Input: part model. Units: mm. Frame: model coordinates. A direction names the side the tool comes from. Round coordinates to 2 decimals unless told otherwise and drop trailing zeros. Write each loop counter-clockwise with the first axis right and the second up, starting at its lowest first coordinate (ties: lowest second). Pieces come first, ordered by that corner, then holes. Notation, with made-up numbers: (27, -12) - (43, -12) arc R27 ccw to (43, 8) - close; hole circle Ø9 at (43, -10). An arc over 180 degrees is marked (long way). Use one line per item in the form item = value.
```python
from build123d import *

# Parameters (mm, degrees)
BOSS_EXTRUDE1_DEPTH     = 60
SKETCH2_W               = 95.474406292
SKETCH2_H               = 38.1
SKETCH2_R               = 1.55
BOSS_EXTRUDE2_DEPTH     = 5.08
SKETCH4_R               = 1.8
CUT_EXTRUDE1_DEPTH      = 96.52
CUT_EXTRUDE1_DEPTH_BACK = 107.696


with BuildPart() as part:
    # Sketch1 → Boss-Extrude1 (new body)
    with BuildSketch(Plane(origin=(0, 0, 0), x_dir=(1, 0, 0), z_dir=(0, 1, 0))):
        with BuildLine():
            Line((-25.4, -19.05), (25.4, -19.05))
            ThreePointArc((25.4, -19.05), (44.45, 0), (25.4, 19.05))
            Line((25.4, 19.05), (-25.4, 19.05))
            ThreePointArc((-25.4, 19.05), (-44.45, 0), (-25.4, -19.05))
        make_face()
        with BuildLine():
            Line((-25.4, -13.97), (25.4, -13.97))
            ThreePointArc((25.4, -13.97), (39.37, 0), (25.4, 13.97))
            Line((25.4, 13.97), (-25.4, 13.97))
            ThreePointArc((-25.4, 13.97), (-39.37, 0), (-25.4, -13.97))
        make_face(mode=Mode.SUBTRACT)
    extrude(amount=BOSS_EXTRUDE1_DEPTH)

    # Sketch2 → Boss-Extrude2 (add)
    with BuildSketch(Plane(origin=(0, 60, 0), x_dir=(1, 0, 0), z_dir=(0, 1, 0))):
        Rectangle(SKETCH2_W, SKETCH2_H)
        with Locations((43.019742204, 15.162081353)):
            Circle(SKETCH2_R, mode=Mode.SUBTRACT)
        with Locations((43.019742204, -15.162081353)):
            Circle(SKETCH2_R, mode=Mode.SUBTRACT)
        with Locations((-43.019742204, -15.162081353)):
            Circle(SKETCH2_R, mode=Mode.SUBTRACT)
        with Locations((-43.019742204, 15.162081353)):
            Circle(SKETCH2_R, mode=Mode.SUBTRACT)
    extrude(amount=-BOSS_EXTRUDE2_DEPTH)

    # Sketch4 → Cut-Extrude1 (cut, two sides)
    with BuildSketch(Plane(origin=(0, 0, 0), x_dir=(0, 0, -1), z_dir=(1, 0, 0))) as cut_extrude1_sk:
        with Locations((0, 5.08)):
            Circle(SKETCH4_R)
    extrude(amount=CUT_EXTRUDE1_DEPTH, mode=Mode.SUBTRACT)
    extrude(cut_extrude1_sk.sketch, amount=-CUT_EXTRUDE1_DEPTH_BACK, mode=Mode.SUBTRACT)


solid = part.part
```
(1) Draft query along Y for faces 1 (the face through (-1, 60, 0)), 2 (the face through (41.815, 3.323, 0.39)), 3 (the face through (-41.815, 3.323, 0.39)), 4 (the face through (44.5, 57.5, 14.7)). Return one class per face: released by +Y, released by -Y, zero draft, split by the parting line, or undercut.
Derived:
face_1 = released by +Y
face_2 = undercut
face_3 = undercut
face_4 = zero draft
(2) Material intervals for L1, parallel to Z at x = -21, y = 43; L2, parallel to X at y = 42, z = 0.5; L3, parallel to Y at x = 16.5, z = 8.5, sorted ascending.
Derived:
L1 = -19.05 to -13.97, 13.97 to 19.05
L2 = -44.44 to -39.36, 39.36 to 44.44
L3 = 54.92 to 60
(3) Cut plane C-C on y = 5.08. Output: boundary loops of the cut face in (x, z).
Derived:
outline = (-44.36, -1.8) arc R19.05 ccw to (-25.4, -19.05) - (25.4, -19.05) arc R19.05 ccw to (44.36, -1.8) - (39.25, -1.8) arc R13.97 cw to (25.4, -13.97) - (-25.4, -13.97) arc R13.97 cw to (-39.25, -1.8) - close; (-44.36, 1.8) - (-39.25, 1.8) arc R13.97 cw to (-25.4, 13.97) - (25.4, 13.97) arc R13.97 cw to (39.25, 1.8) - (44.36, 1.8) arc R19.05 ccw to (25.4, 19.05) - (-25.4, 19.05) arc R19.05 ccw to start
(4) Cut plane D-D on x = 34. Output: boundary loops of the cut face in (y, z).
Derived:
outline = (0, -17) - (54.92, -17) - (54.92, -19.05) - (60, -19.05) - (60, 19.05) - (54.92, 19.05) - (54.92, 17) - (0, 17) - (0, 11.01) - (54.92, 11.01) - (54.92, -11.01) - (0, -11.01) - close
(5) Cut plane A-A on z = 0. Output: boundary loops of the cut face in (x, y), then the cut area to 3 significant figures.
Derived:
outline = (-47.74, 54.92) - (-44.45, 54.92) - (-44.45, 6.88) - (-39.37, 6.88) - (-39.37, 54.92) - (39.37, 54.92) - (39.37, 6.88) - (44.45, 6.88) - (44.45, 54.92) - (47.74, 54.92) - (47.74, 60) - (-47.74, 60) - close; (-44.45, 0) - (-39.37, 0) - (-39.37, 3.28) - (-44.45, 3.28) - close; (39.37, 0) - (44.45, 0) - (44.45, 3.28) - (39.37, 3.28) - close
area = 1,010 mm^2
(6) Access query for faces 5 (the face through (44.445, 27.076, 0.419)), 6 (the face through (39.367, 27.076, 0.307)), 7 (the face through (-45, 54.92, 1)). Directions: +Z, -Z, +X, -X, +Y, -Y. A direction counts if a zero-diameter tool reaches every point of the face in a straight line with its end or side. Return the directions, or none.
Derived:
face_5 = +X, -Y
face_6 = -Y
face_7 = -X, -Y
(7) First-contact query: pin 1 Ø3 at (x, z) = (43.02, -15.16) entering from -Y; pin 2 Ø8.5 at (x, z) = (-14.5, -3) entering from -Y; pin 3 Ø1.5 at (y, z) = (11, -4.5) entering from +X; pin 4 Ø4 at (y, z) = (5.08, 0) entering from -X. Flat tips, straight axial feed; report the tip coordinate or a pass-through.
Derived:
pin_1 = through
pin_2 = 54.92
pin_3 = 44.08
pin_4 = -44.45
(8) Cut plane B-B on y = 41. Output: boundary loops of the cut face in (x, z).
Derived:
outline = (-25.4, -19.05) - (25.4, -19.05) arc R19.05 ccw to (25.4, 19.05) - (-25.4, 19.05) arc R19.05 ccw to start; hole (-25.4, -13.97) - (25.4, -13.97) arc R13.97 ccw to (25.4, 13.97) - (-25.4, 13.97) arc R13.97 ccw to start
